Autodesk Fusion 360 part; units mm, degrees
sketch "Base" plane through (0, 0, 0) normal (0, 0, 1) x (1, 0, 0)
  circle A0 centre (0, 0) radius 30
  circle A1 centre (0, 0) radius 28
  dimension "d1" = 60
  dimension "d2" = 56
extrude "Extrude1" add sketch "Base" along normal blind 2 contours A1 makes body 1
extrude "Extrude2" add sketch "Base" along normal blind 113 bodies 1
sketch "Sketch2" plane through (0, 0, 0) normal (0, 0, 1) x (1, 0, 0)
  circle A0 centre (0, 0) radius 28
  line L0 (0, -2) -> (27.9285, -2)
  line L1 (-27.9285, -2) -> (0, -2)
  line L2 (0, 2) -> (-27.9285, 2)
  line L3 (27.9285, 2) -> (0, 2)
  circle A1 centre (0, 0) radius 30
extrude "Extrude3" add sketch "Sketch2" along normal blind 3 separate body makes body 2
extrude "Extrude4" add sketch "Sketch2" along normal blind 5 contours A0 L0 L1 bodies 2
extrude "Extrude5" add sketch "Sketch2" along normal blind 5 contours A0 L2 L3 bodies 2
extrude "Extrude6" add sketch "Sketch2" along normal blind 110 contours A0 L0 L1 L2 L3 bodies 2
sketch "Sketch6" plane through (0, 2, 0) normal (0, 1, 0) x (-1, 0, 0)
  line L0 (-27.9285, 5) -> (27.9285, 5)
  line L1 (27.9285, 5) -> (27.9285, 110)
  line L2 (27.9285, 110) -> (-27.9285, 110)
  line L3 (-27.9285, 110) -> (-27.9285, 5)
  line L4 (-2.5, 7.5) -> (2.5, 7.5)
  line L5 (2.5, 7.5) -> (2.5, 110)
  line L6 (-2.5, 110) -> (2.5, 110)
  line L7 (-2.5, 110) -> (-2.5, 7.5)
  dimension "d15" = 102.5
  dimension "d16" = 5
extrude "Extrude7" cut sketch "Sketch6" against normal blind 4 contours L2 L4 L5 L6 L7 bodies 2
sketch "Sketch7" plane through (0, 0, 0) normal (0, 0, 1) x (1, 0, 0)
  circle A0 centre (-100, 0) radius 30
  circle A1 centre (-100, 0) radius 28
  line L0 (-100, 5) -> (-72.45, 5)
  line L1 (-100, -5) -> (-72.45, -5)
  line L2 (-100, -5) -> (-127.55, -5)
  line L3 (-100, 5) -> (-127.55, 5)
  line L4 (-100, -7) -> (-72.8891, -7)
  line L5 (-100, -7) -> (-127.1109, -7)
  line L6 (-100, 7) -> (-72.8891, 7)
  line L7 (-100, 7) -> (-127.1109, 7)
extrude "Extrude8" add sketch "Sketch7" along normal blind 3 separate body makes body 3
extrude "Extrude9" add sketch "Sketch7" along normal blind 5 contours A1 L6 L7 bodies 3
extrude "Extrude10" add sketch "Sketch7" along normal blind 5 contours A1 L0 L1 L2 L3 bodies 3
extrude "Extrude11" add sketch "Sketch7" along normal blind 5 contours A1 L4 L5 bodies 3
extrude "Extrude12" add sketch "Sketch7" along normal blind 110 contours A1 L0 L3 L6 L7 bodies 3
extrude "Extrude13" add sketch "Sketch7" along normal blind 110 contours A1 L1 L2 L4 L5 bodies 3
sketch "Sketch8" plane through (0, -7, 0) normal (0, -1, 0) x (1, 0, 0)
  line L0 (-127.1109, 5) -> (-72.8891, 5)
  line L1 (-72.8891, 5) -> (-72.8891, 110)
  line L2 (-72.8891, 110) -> (-127.1109, 110)
  line L3 (-127.1109, 110) -> (-127.1109, 5)
  line L4 (-102, 10) -> (-98, 10)
  line L5 (-98, 10) -> (-98, 110)
  line L6 (-102, 10) -> (-102, 110)
extrude "Extrude14" cut sketch "Sketch8" against normal blind 200 contours L2 L4 L5 L6 bodies 3
hidden bodies 1 2
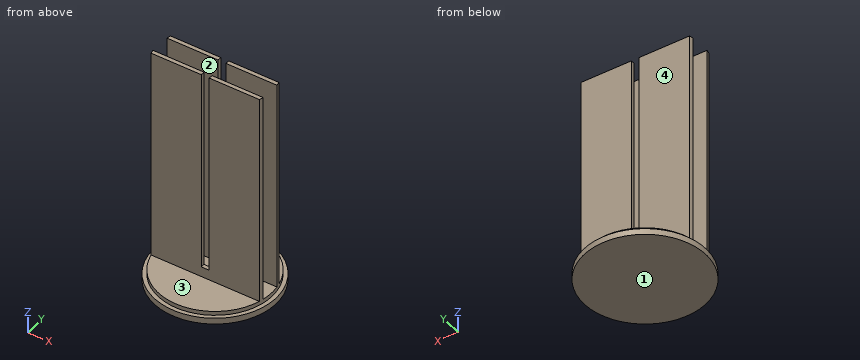
Check sheet for the modelled part. Datum: model origin and axes. Units: mm. Face numbers are marked on the shaded views. A direction names the side the tool comes from. Round coordinates to 2 decimals unless told otherwise and drop trailing zeros. Order: outer loops, then holes, each group sorted by start corner. A loop starts at its lowest first (then second) coordinate and runs counter-clockwise, first axis right, second up. Notation, with made-up numbers: (-39.5, 88.5) -> (4.5, 88.5) arc R29 cw to (4.5, 108.5) -> close; hole circle Ø9 at (25.25, -1). An arc over 180 degrees is marked (long way). One line per item, written item: value. Start each with the question number.
Q1. Cross-section at B-B (z = 27.5). Record the boundary of the cut face in (x, y), and give its area (3 significant figures).
Q2. Cross-section at C-C (y = 0). Record the boundary of the cut face in (x, z), and give its area (3 significant figures).
Q3. Set-up check for the marked faces 1, 2, 3 and 4: record each of +Z, -Z, +X, -X, +Y, -Y from which the full face is reachable in a straight line by a thin tool's end or side.
Q4. Cross-section at A-A (x = -100). Record the boundary of the cut face in (y, z), and give its area (3 significant figures).
Q5. Gauge pin test, flat ends, axial feed: pin 1 Ø1.6 at (x, y) = (-99.5, -6) entering from +Z; pin 2 Ø6 at (y, z) = (-7.5, 83) entering from -X; pin 3 Ø3 at (x, y) = (-100.5, -0.5) entering from +Z. Record the tip position at first contact, or that the pin passes through.
Q6. Cross-section at D-D (x = -119.5). Record the boundary of the cut face in (y, z), and give its area (3 significant figures).
Q7. Thickness scan on line 1 (Y direction, x = -76.5, z = 95); line 2 (Z direction, x = -79.5, y = -8); line 3 (X direction, y = 6.5, z = 7). Record the ranges inside material, lowest first.
Completed:
1. outline: (-127.55, -5) arc R28 ccw to (-127.11, -7) -> (-102, -7) -> (-102, -5) -> close; (-127.55, 5) -> (-102, 5) -> (-102, 7) -> (-127.11, 7) arc R28 ccw to start; (-98, -7) -> (-72.89, -7) arc R28 ccw to (-72.45, -5) -> (-98, -5) -> close; (-98, 5) -> (-72.45, 5) arc R28 ccw to (-72.89, 7) -> (-98, 7) -> close
1. area: 203 mm²
2. outline: (-130, 0) -> (-70, 0) -> (-70, 3) -> (-72, 3) -> (-72, 5) -> (-128, 5) -> (-128, 3) -> (-130, 3) -> close
2. area: 292 mm²
3. face 1: -Z, +X, -X, +Y, -Y
3. face 2: +Z, +X, -X
3. face 3: +Z, +X, -X, -Y
3. face 4: +Z, +X, -X, +Y
4. outline: (-30, 0) -> (30, 0) -> (30, 3) -> (28, 3) -> (28, 5) -> (7, 5) -> (7, 10) -> (5, 10) -> (5, 5) -> (-5, 5) -> (-5, 10) -> (-7, 10) -> (-7, 5) -> (-28, 5) -> (-28, 3) -> (-30, 3) -> close
4. area: 312 mm²
5. pin 1: stops at z = 10
5. pin 2: stops at x = -127.55
5. pin 3: stops at z = 5
6. outline: (-22.8, 0) -> (22.8, 0) -> (22.8, 3) -> (20.09, 3) -> (20.09, 5) -> (7, 5) -> (7, 110) -> (5, 110) -> (5, 5) -> (-5, 5) -> (-5, 110) -> (-7, 110) -> (-7, 5) -> (-20.09, 5) -> (-20.09, 3) -> (-22.8, 3) -> close
6. area: 637 mm²
7. line 1: y = -7 to -5, 5 to 7
7. line 2: z = 0 to 5
7. line 3: x = -127.24 to -72.76
